```python
from build123d import *

# Parameters (mm, degrees)
SKETCH1_W           = 5
SKETCH1_H           = 7
BOSS_EXTRUDE1_DEPTH = 4.5
SKETCH2_W           = 0.284935897
SKETCH2_H           = 3.175
CUT_EXTRUDE1_DEPTH  = 1.27


with BuildPart() as part:
    # Sketch1 → Boss-Extrude1 (new body)
    with BuildSketch(Plane.XY):
        with Locations((2.5, 3.5)):
            Rectangle(SKETCH1_W, SKETCH1_H)
    extrude(amount=BOSS_EXTRUDE1_DEPTH)

    # Sketch2 → Cut-Extrude1 (cut)
    # profile 1 of 2: a face of its own
    with BuildSketch(Plane.XY.offset(4.5)):
        with Locations((1.019007648, 4.325358418)):
            Rectangle(SKETCH2_W, SKETCH2_H)
    # profile 2 of 2: a face of its own
    with BuildSketch(Plane.XY.offset(4.5)):
        with BuildLine():
            Line((1.97557816, 5.912858418), (2.610959771, 5.912858418))
            add(Edge.make_bspline(
                [(2.610959771, 5.912858418), (2.653360651, 5.91271728), (2.73477504, 5.912446278), (2.851409363, 5.910935193), (2.95738823, 5.90660417), (3.052656227, 5.902877098), (3.137211607, 5.896080837), (3.211313649, 5.889585107), (3.274621061, 5.881081858), (3.312944083, 5.873184795), (3.330295708, 5.86960922)],
                knots=[0, 0, 0, 0, 1.410062039, 2.707475311, 3.878576406, 4.937260626, 5.877586885, 6.699081471, 7.410979367, 8, 8, 8, 8], degree=3))
            add(Edge.make_bspline(
                [(3.330295708, 5.86960922), (3.353524574, 5.86386994), (3.399486772, 5.852513814), (3.465662903, 5.828511176), (3.528722326, 5.800734802), (3.588403095, 5.76811057), (3.644406277, 5.730396306), (3.697309316, 5.688243081), (3.747352272, 5.641881544), (3.792511322, 5.590142795), (3.835091748, 5.535862532), (3.871004287, 5.477166982), (3.90196188, 5.41578831), (3.92660942, 5.351102296), (3.946455868, 5.28373626), (3.96044967, 5.213079994), (3.968841819, 5.139455395), (3.969696217, 5.089237864), (3.970129442, 5.063774885)],
                knots=[0, 0, 0, 0, 1.027469482, 2.033020251, 3.019912614, 3.986113645, 4.951240523, 5.91722682, 6.890402269, 7.87763091, 8.8651537, 9.85103654, 10.82876324, 11.815024772, 12.821070561, 13.842952187, 14.906261191, 16, 16, 16, 16], degree=3))
            add(Edge.make_bspline(
                [(3.970129442, 5.063774885), (3.968796851, 5.021470183), (3.96619662, 4.938922752), (3.941953134, 4.819124667), (3.902241576, 4.70737436), (3.847519736, 4.603812538), (3.777833497, 4.510457881), (3.694081722, 4.428460825), (3.596217689, 4.359844619), (3.505113952, 4.312262432), (3.4246375, 4.281788865), (3.358385852, 4.260347311), (3.286116522, 4.243781099), (3.20852194, 4.228940123), (3.125279195, 4.217735371), (3.036587802, 4.209528818), (2.942384508, 4.204399788), (2.877669781, 4.203635969), (2.84437824, 4.203243034)],
                knots=[0, 0, 0, 0, 1.260483769, 2.459530307, 3.627416485, 4.787058657, 5.939039949, 7.08810263, 8.267026773, 9.491475466, 10.141966685, 10.831826277, 11.566392101, 12.351337768, 13.187381173, 14.07005841, 15.007169909, 16, 16, 16, 16], degree=3))
            Line((2.84437824, 4.203243034), (4.01083457, 2.737858418))
            Line((4.01083457, 2.737858418), (3.658480804, 2.737858418))
            Line((3.658480804, 2.737858418), (2.492024474, 4.203243034))
            Line((2.492024474, 4.203243034), (2.260514057, 4.203243034))
            Line((2.260514057, 4.203243034), (2.260514057, 2.737858418))
            Line((2.260514057, 2.737858418), (1.97557816, 2.737858418))
            Line((1.97557816, 2.737858418), (1.97557816, 5.912858418))
        make_face()
        with BuildLine():
            Line((2.260514057, 5.587217393), (2.260514057, 4.528884059))
            Line((2.260514057, 4.528884059), (2.84183417, 4.524431936))
            add(Edge.make_bspline(
                [(2.84183417, 4.524431936), (2.868975919, 4.524419928), (2.92158436, 4.524396654), (2.997694249, 4.52801958), (3.06856035, 4.532141019), (3.133911604, 4.538445068), (3.193777205, 4.546569504), (3.24812723, 4.556732211), (3.297050398, 4.568572297), (3.354108358, 4.586898057), (3.417822926, 4.615932088), (3.487066464, 4.658173648), (3.546032871, 4.711304206), (3.595851217, 4.772058698), (3.635882916, 4.838857295), (3.664105994, 4.910899287), (3.682015209, 4.986365951), (3.684127532, 5.038234663), (3.685193545, 5.064410902)],
                knots=[0, 0, 0, 0, 1.146690395, 2.22261258, 3.21895312, 4.145990853, 4.996080663, 5.770904154, 6.481378293, 7.121626537, 8.300444488, 9.431385265, 10.535395872, 11.636531494, 12.74115979, 13.810798291, 14.895190096, 16, 16, 16, 16], degree=3))
            add(Edge.make_bspline(
                [(3.685193545, 5.064410902), (3.684103049, 5.089943866), (3.681942085, 5.140540882), (3.664299273, 5.214614458), (3.634463906, 5.284525191), (3.594257304, 5.349988688), (3.545272357, 5.409411749), (3.487834055, 5.460254523), (3.423512914, 5.502209395), (3.36339547, 5.52901944), (3.309661577, 5.545456735), (3.263007528, 5.557023863), (3.210292116, 5.566317059), (3.151259379, 5.573762943), (3.086161328, 5.580162785), (3.014668809, 5.584473328), (2.937256158, 5.587025904), (2.883601442, 5.587152078), (2.855826557, 5.587217393)],
                knots=[0, 0, 0, 0, 1.101028733, 2.181837193, 3.264309656, 4.369019818, 5.486613113, 6.575447106, 7.666700264, 8.788928104, 9.402425223, 10.0903467, 10.862060571, 11.710948788, 12.657782767, 13.684531032, 14.801375019, 16, 16, 16, 16], degree=3))
            Line((2.855826557, 5.587217393), (2.260514057, 5.587217393))
        make_face(mode=Mode.SUBTRACT)
    extrude(amount=-CUT_EXTRUDE1_DEPTH, mode=Mode.SUBTRACT)


solid = part.part
```
The listing builds one solid part. Answer for the finished solid, in the listing's coordinates (mm). A direction names the side the tool comes from. Coordinates: 2 decimals unless noted, no trailing zeros. Write item = value, one per line.
1) Which of the six approach directions +Z, -Z, +X, -X, +Y, -Y give full straight-line access (tool end or side, diameter ignored) to faces 1 (the face through (1.976, 4, 4)), 2 (the face through (2, 4, 0))?
Responses:
face_1 = +Z
face_2 = -Z, +X, -X, +Y, -Y
2) Determine the mould class of faces 3 (the face through (2.261, 5, 4)), 4 (the face through (3, 5, 4.5)), 5 (the face through (0, 3, 2)), 6 (the face through (2.261, 3, 4)) for opening direction X: pulls with the +X half, pulls with the -X half, needs draft (parallel to the pull), parting line crosses it, or undercut.
Responses:
face_3 = undercut
face_4 = needs draft
face_5 = pulls with the -X half
face_6 = undercut
3) Section A-A (z = 3.5) is taken. Count the separate pieces of the cut face and the enclosed holes in it, plus the area to 3 significant figures.
Responses:
separate_pieces = 2
enclosed_holes = 2
area = 31.5 mm^2
4) Find the intervals of material crossed by line 1 along X through (y, z) = (4.75, 3.85); line 2 along X through (y, z) = (3.75, 4.1); line 3 along Y through (x, z) = (3.35, 4.1), in increasing order.
Responses:
line_1 = 0 to 0.88, 1.16 to 1.98, 2.26 to 3.58, 3.92 to 5
line_2 = 0 to 0.88, 1.16 to 1.98, 2.26 to 2.85, 3.21 to 5
line_3 = 0 to 3.13, 3.57 to 4.26, 4.59 to 5.53, 5.86 to 7
